The listing builds one solid part. Answer for the finished solid, in the listing's coordinates (mm). A direction names the side the tool comes from. Round coordinates to 2 decimals unless told otherwise and drop trailing zeros. Write each loop counter-clockwise with the first axis right and the second up, starting at its lowest first coordinate (ties: lowest second). Pieces come first, ordered by that corner, then holes. Notation, with made-up numbers: M 63.5,-0.75 L 121.5,-0.75 A26 ccw 121.5,23.25 Z; hole C -9.75,58 d11. An arc over 180 degrees is marked long. Write each question's results on one line, items separated by ' | '.
from build123d import *

# Parameters (mm, degrees)
SKETCH_1_W      = 6
SKETCH_1_H      = 4
EXTRUDE_1_DEPTH = 7
SKETCH_2_R      = 2.5
EXTRUDE_2_DEPTH = 2
FILLET_1_R      = 2.5
SKETCH_3_W      = 1
SKETCH_3_H      = 0.5


with BuildPart() as part:
    # 草图1 → 拉伸1 (new body)
    with BuildSketch(Plane(origin=(0, 0, 0), x_dir=(1, 0, 0), z_dir=(0, 1, 0))):
        Rectangle(SKETCH_1_W, SKETCH_1_H)
    extrude(amount=EXTRUDE_1_DEPTH)

    # 草图2 → 拉伸2 (add)
    with BuildSketch(Plane(origin=(0, 0, -2), x_dir=(-1, 0, 0), z_dir=(0, 0, -1))):
        with Locations(Location((0, 4.040945029, 0), (0, 0, 180))):
            Circle(SKETCH_2_R)
    extrude(amount=EXTRUDE_2_DEPTH)

    # 圆角1
    # the kernel refuses this fillet: 2.5 mm, written as the material it takes off along each edge
    with BuildSketch(Plane(origin=(0, 4.040945029, -4), x_dir=(1, 0, 0), z_dir=(0, 1, 0))) as fillet_1_piece_1:
        with BuildLine():
            CenterArc((0.050510257, -2.5), FILLET_1_R, 11.536959033, 78.463040967)
            Line((0.050510257, 0), (0.050510257, 0.05))
            Line((0.050510257, 0.05), (2.5, 0.05))
            Line((2.5, 0.05), (2.55, 0))
            ThreePointArc((2.55, 0), (2.55, -1), (2.548989795, -1.99))
            Line((2.548989795, -1.99), (2.5, -2))
        make_face()
    revolve(axis=Axis((0, 4.040945029, -4), (0, 0, -1)), mode=Mode.SUBTRACT)

    # 扫描1: sweep along a path in 草图4
    with BuildLine(Plane(origin=(0, 0, 0), x_dir=(0, 0, -1), z_dir=(1, 0, 0))) as sweep_1_path:
        Line((0, 0), (0, -1))
        ThreePointArc((0, -1), (-0.292893219, -1.707106781), (-1, -2))
        Line((-1, -2), (-13.273282855, -2))
    # 草图3 → 扫描1 (sweep)
    with BuildSketch(Plane.XZ):
        Rectangle(SKETCH_3_W, SKETCH_3_H)
        with Locations((2.54, 0)):
            Rectangle(SKETCH_3_W, SKETCH_3_H)
        with Locations((-2.54, 0)):
            Rectangle(SKETCH_3_W, SKETCH_3_H)
    sweep(path=sweep_1_path.line)


solid = part.part
1) Find the intervals of material crossed by line 1 (Z direction, x = -0.75, y = 1); line 2 (Y direction, x = 1.75, z = -0.75); line 3 (Z direction, x = 0.75, y = 4.25), in increasing order.
Return value:
line 1: -2 to 2 | line 2: 0 to 7 | line 3: -3.89 to 2
2) The mould has two halves that part along Y. Classify faces 4 (the face through (0, 7, 0)), 5 (the face through (0, -2.25, 7)), 6 (the face through (3.04, -2, 6)), 7 (the face through (0, -0.5, 0.25)): +Y half, -Y half, draft (parallel to the pull), parting line (faces both ways), or undercut.
Return value:
face 4: +Y half | face 5: -Y half | face 6: draft | face 7: undercut
3) A tool of negligible diameter and unlimited length cuts with its end or side. For faces 1 (the face through (2.5, -0.5, 0.25)), 2 (the face through (0.5, -2, 6)), 3 (the face through (0, 3, 2)), from which of +Z, -Z, +X, -X, +Y, -Y can it reach the whole face along a straight path? Write none if from no direction.
Return value:
face 1: +Z, +X, -X | face 2: +Z, -Z, -Y | face 3: +Z, +X, -X, +Y
4) Section A-A (z = 10) is taken. Determine the outline of the cut face in (x, y).
Return value:
outline: M -3.04,-2.25 L -2.04,-2.25 L -2.04,-1.75 L -3.04,-1.75 Z; M -0.5,-2.25 L 0.5,-2.25 L 0.5,-1.75 L -0.5,-1.75 Z; M 2.04,-2.25 L 3.04,-2.25 L 3.04,-1.75 L 2.04,-1.75 Z
5) Each of these flat-tipped pins is pushed along its axis until it touches: pin 1 (0.5 mm diameter, centred on x = 0, z = 8.5, fed in from +Y); pin 2 (2 mm diameter, centred on y = 4.5, z = -0.5, fed in from -X); pin 3 (2 mm diameter, centred on y = 4, z = 0, fed in from +X); pin 4 (1.1 mm diameter, centred on y = -0.5, z = 8.5, fed in from -X). Where does it stop, or does it pass through?
Return value:
pin 1: y = -1.75 | pin 2: x = -3 | pin 3: x = 3 | pin 4: through
6) Section B-B (y = -1.5) is taken. Determine the outline of the cut face in (x, z).
Return value:
outline: M -3.04,-0.15 L -2.04,-0.15 L -2.04,0.44 L -3.04,0.44 Z; M -0.5,-0.15 L 0.5,-0.15 L 0.5,0.44 L -0.5,0.44 Z; M 2.04,-0.15 L 3.04,-0.15 L 3.04,0.44 L 2.04,0.44 Z
